Read the model definition and answer for the solid it produces. Units are mm, in the model's axes. Face numbers are marked on the shaded views. A direction names the side the tool comes from. Coordinates: 2 decimals unless noted, no trailing zeros. Write each loop counter-clockwise with the first axis right and the second up, starting at its lowest first coordinate (ties: lowest second). Pieces come first, ordered by that corner, then holes. Notation, with made-up numbers: (1.5, 73) -> (15.5, 73) arc R32 cw to (15.5, 99) -> close; hole circle Ø3 at (42.25, -13.5). An arc over 180 degrees is marked (long way). Answer in a Markdown table with one row per item. Add a question column.
Item 1: Section D-D on z = 6.5 is taken. Write down the section's boundary in (x, y).
Item 2: Section A-A on z = 10.25 is taken. Write down the section's boundary in (x, y).
Item 3: For a pull along X with two mould halves and no side action, classify the marked faces 4, 5, 6 and 7 as +X half, -X half, draft (parallel to the pull), parting line (faces both ways), or undercut.
Item 4: Section C-C on y = 12 is taken. Write down the section's boundary in (x, z), then the cut area to 3 significant figures.
Item 5: Section B-B on x = 3.75 is taken. Write down the section's boundary in (y, z).
Item 6: Straight lines are drawn through the part: line 1 (Z direction, x = 4, y = 12.25); line 2 (X direction, y = 1.4, z = 10.25); line 3 (Y direction, x = -3.5, z = 11.5). For each, find the intervals that lie inside material, in ascending order. Write a range as from..to.
Item 7: Which of the six approach directions +Z, -Z, +X, -X, +Y, -Y give full straight-line access (tool end or side, diameter ignored) to the marked faces 1, 2 and 3?
Item 8: Given pin 1 Ø3 at (x, z) = (-26, 20.5) entering from -Y; pin 2 Ø1.5 at (x, z) = (-9, 9.5) entering from +Y; pin 3 Ø2 at (x, z) = (-13, 10.5) entering from -Y; pin 4 Ø2 at (x, y) = (3, 9) entering from -Z, each flat-ended and moving along its own axis, determine where each tip first touches the part or whether it passes through.
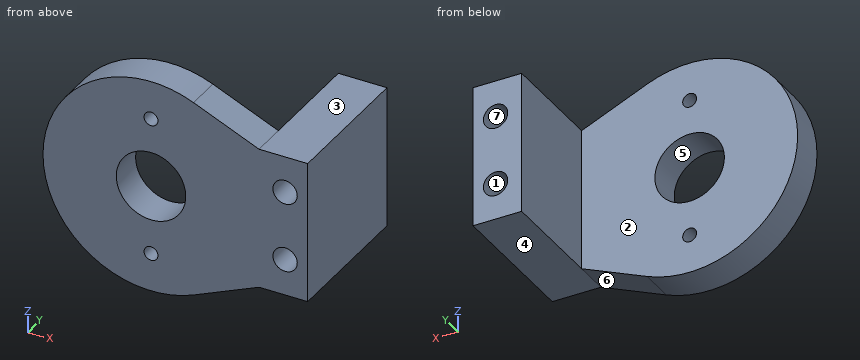
```python
from build123d import *

# Parameters (mm, degrees)
SKETCH1_W               = 7
SKETCH1_H               = 20.5
MOUNTINGBASE_DEPTH      = 20.50030868
SKETCH2_R               = 1.75
MOUNTINGHOLES_DEPTH     = 30.824698757
HORNTAB_DEPTH           = 5
SKETCH4_R               = 1
SKETCH4_R_2             = 5
HORNMOUNTINGHOLES_DEPTH = 5


with BuildPart() as part:
    # Sketch1 → mountingBase (new body)
    with BuildSketch(Plane(origin=(0, 0, 0), x_dir=(1, 0, 0), z_dir=(0, 1, 0))):
        with Locations((3.5, -10.25)):
            Rectangle(SKETCH1_W, SKETCH1_H)
    extrude(amount=MOUNTINGBASE_DEPTH)

    # Sketch2 → mountingHoles (cut, through all)
    with BuildSketch(Plane(origin=(0, 20.50030868, 0), x_dir=(1, 0, 0), z_dir=(0, 1, 0))):
        with Locations(Location((3.75, -5.25, 0), (0, 0, 270))):
            Circle(SKETCH2_R)
        with Locations(Location((3.75, -15.25, 0), (0, 0, 90))):
            Circle(SKETCH2_R)
    extrude(amount=-MOUNTINGHOLES_DEPTH, mode=Mode.SUBTRACT)

    # Sketch3 → hornTab (add)
    with BuildSketch(Plane(origin=(0, 0, 0), x_dir=(1, 0, 0), z_dir=(0, 1, 0))):
        with BuildLine():
            Line((0, 0), (-9.422358224, 4.035054584))
            ThreePointArc((-9.422358224, 4.035054584), (-31.07965246, -10.25), (-9.422358224, -24.535054584))
            Line((-9.422358224, -24.535054584), (0, -20.5))
            Line((0, -20.5), (0, 0))
        make_face()
    extrude(amount=HORNTAB_DEPTH)

    # Sketch4 → hornMountingHoles (cut)
    with BuildSketch(Plane(origin=(0, 5, 0), x_dir=(1, 0, 0), z_dir=(0, 1, 0))):
        with Locations(Location((-15.53982623, -0.25, 0), (0, 0, 270))):
            Circle(SKETCH4_R)
        with Locations(Location((-15.53982623, -20.25, 0), (0, 0, 90))):
            Circle(SKETCH4_R)
        with Locations(Location((-15.53982623, -10.25, 0), (0, 0, 270))):
            Circle(SKETCH4_R_2)
    extrude(amount=-HORNMOUNTINGHOLES_DEPTH, mode=Mode.SUBTRACT)


solid = part.part
```
Results below:
| question | item | result |
|---|---|---|
| 1 | outline | (-30.62, 0) -> (-18.85, 0) -> (-18.85, 5) -> (-30.62, 5) -> close; (-12.23, 0) -> (2.53, 0) -> (2.53, 20.5) -> (0, 20.5) -> (0, 5) -> (-12.23, 5) -> close; (4.97, 0) -> (7, 0) -> (7, 20.5) -> (4.97, 20.5) -> close |
| 2 | outline | (-31.08, 0) -> (-20.54, 0) -> (-20.54, 5) -> (-31.08, 5) -> close; (-10.54, 0) -> (7, 0) -> (7, 20.5) -> (0, 20.5) -> (0, 5) -> (-10.54, 5) -> close |
| 3 | face 4 | draft |
| 3 | face 5 | undercut |
| 3 | face 6 | +X half |
| 3 | face 7 | undercut |
| 4 | outline | (0, 0) -> (7, 0) -> (7, 20.5) -> (0, 20.5) -> close; hole circle Ø3.5 at (3.75, 5.25); hole circle Ø3.5 at (3.75, 15.25) |
| 4 | area | 124 mm2 |
| 5 | outline | (0, 0) -> (20.5, 0) -> (20.5, 3.5) -> (0, 3.5) -> close; (0, 7) -> (20.5, 7) -> (20.5, 13.5) -> (0, 13.5) -> close; (0, 17) -> (20.5, 17) -> (20.5, 20.5) -> (0, 20.5) -> close |
| 6 | line 1 | z = 0..3.52, 6.98..13.52, 16.98..20.5 |
| 6 | line 2 | x = -31.08..-20.54, -10.54..7 |
| 6 | line 3 | y = 0..5 |
| 7 | face 1 | +Y, -Y |
| 7 | face 2 | +Z, -Z, -X, +Y |
| 7 | face 3 | +Z, +X, +Y, -Y |
| 8 | pin 1 | stops at y = 0 |
| 8 | pin 2 | stops at y = 5 |
| 8 | pin 3 | passes through |
| 8 | pin 4 | stops at z = 0 |
